Can you work these out from the model? Positions are in its coordinate system, mm. A direction names the side the tool comes from. Coordinates: 2 decimals unless noted, no trailing zeros. Order: outer loops, then holes, each group sorted by start corner. A loop starts at its lowest first (then second) coordinate and runs counter-clockwise, first axis right, second up.
```python
from build123d import *

# Parameters (mm, degrees)
BOSS_EXTRUDE1_DEPTH      = 5.588
BOSS_EXTRUDE1_DEPTH_BACK = 2.54


with BuildPart() as part:
    # Sketch1 → Boss-Extrude1 (new, two sides: drawn at the far end of the back side and taken through both)
    with BuildSketch(Plane(origin=(0, 0, 0), x_dir=(1, 0, 0), z_dir=(0, 1, 0)).offset(-BOSS_EXTRUDE1_DEPTH_BACK)):
        with BuildLine():
            Line((-49.445827732, 34.925), (-25.939086815, 1.353894815))
            ThreePointArc((-25.939086815, 1.353894815), (-24.804330922, 0.358740605), (-23.338279075, 0))
            Line((-23.338279075, 0), (23.338279075, 0))
            ThreePointArc((23.338279075, 0), (24.804330922, 0.358740605), (25.939086815, 1.353894815))
            Line((25.939086815, 1.353894815), (49.445827732, 34.925))
            Line((49.445827732, 34.925), (52.046635473, 33.103894815))
            Line((52.046635473, 33.103894815), (28.539894556, -0.467210371))
            ThreePointArc((28.539894556, -0.467210371), (26.270382769, -2.457518791), (23.338279075, -3.175))
            Line((23.338279075, -3.175), (-23.338279075, -3.175))
            ThreePointArc((-23.338279075, -3.175), (-26.270382769, -2.457518791), (-28.539894556, -0.467210371))
            Line((-28.539894556, -0.467210371), (-52.046635473, 33.103894815))
            Line((-52.046635473, 33.103894815), (-49.445827732, 34.925))
        make_face()
    extrude(amount=BOSS_EXTRUDE1_DEPTH + BOSS_EXTRUDE1_DEPTH_BACK)


solid = part.part
```
1. Imagine slicing it at D-D on x = 25. Please give me the cut outline in (y, z), then the cut area to 3 significant figures.
Completed:
outline: (-2.54, -0.47) - (5.59, -0.47) - (5.59, 2.95) - (-2.54, 2.95) - close
area: 27.8 mm2
2. I'm going to push flat-ended pins straight in: pin 1 (2.5 mm diameter, centred on x = 11.5, y = 1.5, fed in from -Z); pin 2 (1 mm diameter, centred on x = -30, y = 3, fed in from +Z); pin 3 (12 mm diameter, centred on x = -41.5, z = -2, fed in from +Y). Where does each tip first touch, or does it pass through?
Completed:
pin 1: stops at z = 0
pin 2: stops at z = -0.9
pin 3: passes through
3. On a 3-axis mill with a long thin cutter (end or side, diameter ignored), from which of +Z, -Z, +X, -X, +Y, -Y can I reach the whole of each face in a straight line? I mean faces 4 (the cylindrical face through (24.79, 1.47, -0.35)), 5 (the cylindrical face through (-26.23, 1.47, 2.48)). Say none if no direction works.
Completed:
face 4: -Z, +Y, -Y
face 5: +Z, -X, +Y, -Y
4. Imagine slicing it at A-A on y = 3. Please give me the cut outline in (x, z) (3 decimals).
Completed:
outline: (-52.047, -33.104) - (-49.446, -34.925) - (-25.939, -1.354) arc R3.175 cw to (-23.338, 0) - (23.338, 0) arc R3.175 cw to (25.939, -1.354) - (49.446, -34.925) - (52.047, -33.104) - (28.54, 0.467) arc R6.35 ccw to (23.338, 3.175) - (-23.338, 3.175) arc R6.35 ccw to (-28.54, 0.467) - close
5. Imagine slicing it at C-C on x = 3. Please give me the cut outline in (y, z) (3 decimals).
Completed:
outline: (-2.54, 0) - (5.588, 0) - (5.588, 3.175) - (-2.54, 3.175) - close
6. Thinking about a two-plate mould opening in X: for faces 1 (the flat face through (37.528, 1.467, -17.904)), 2 (the flat face through (0, 5.588, 1)), 3 (the flat face through (40.458, 1.467, -16.553)), which applies, pulls with the +X half, pulls with the -X half, needs draft (parallel to the pull), parting line crosses it, or undercut?
Completed:
face 1: undercut
face 2: needs draft
face 3: pulls with the +X half
7. Imagine slicing it at B-B on z = -30. Please give me the cut outline in (x, y), then the cut area to 3 significant figures.
Completed:
outline: (-49.87, -2.54) - (-46, -2.54) - (-46, 5.59) - (-49.87, 5.59) - close; (46, -2.54) - (49.87, -2.54) - (49.87, 5.59) - (46, 5.59) - close
area: 63.0 mm2
8. Please list where these lines run through material, in increasing order: probe 1 along Z at (x, y) = (-17, 5.25) (3 decimals); probe 2 along X at (y, z) = (-2, -32); probe 3 along X at (y, z) = (2.5, -16.5).
Completed:
probe 1: z = 0 to 3.175
probe 2: x = -51.27 to -47.4, 47.4 to 51.27
probe 3: x = -40.42 to -36.54, 36.54 to 40.42
